from build123d import *

# Parameters (mm, degrees)
SKETCH1_W           = 300
SKETCH1_H           = 300
SKETCH1_W_2         = 350
BOSS_EXTRUDE1_DEPTH = 5
SKETCH2_W           = 50
SKETCH2_H           = 50
BOSS_EXTRUDE2_DEPTH = 75


with BuildPart() as part:
    # Sketch1 → Boss-Extrude1 (new body, symmetric)
    with BuildSketch(Plane(origin=(0, 0, 0), x_dir=(1, 0, 0), z_dir=(0, 1, 0))):
        Rectangle(SKETCH1_W, SKETCH1_H)
        with Locations((325, 0)):
            Rectangle(SKETCH1_W_2, SKETCH1_H)
    extrude(amount=BOSS_EXTRUDE1_DEPTH, both=True)

    # Sketch2 → Boss-Extrude2 (add)
    with BuildSketch(Plane(origin=(0, 5, 0), x_dir=(1, 0, 0), z_dir=(0, 1, 0))):
        with Locations((435, 0)):
            Rectangle(SKETCH2_W, SKETCH2_H)
    extrude(amount=BOSS_EXTRUDE2_DEPTH)


solid = part.part
CAD build for the part. Positions are in the model's coordinates, mm. A direction names the side the tool comes from. Coordinates: 2 decimals unless noted, no trailing zeros. Loops run counter-clockwise (first coordinate to the right, second up) from the corner with the lowest first, then second, coordinate; pieces in that order, holes last. Notation, with made-up numbers: (-4, 83) -> (44, 83) arc R21 ccw to (44, 109) -> close; hole circle Ø3 at (2, -25). An arc over 180 degrees is marked (long way). One line per item, written item: value.
1. Slice it at A-A on z = 2.5. Write the cut outline in (x, y), and give its area (4 significant figures).
Answers:
outline: (-150, -5) -> (500, -5) -> (500, 5) -> (460, 5) -> (460, 80) -> (410, 80) -> (410, 5) -> (-150, 5) -> close
area: 10,250 mm^2
2. Slice it at C-C on y = 29. Write the cut outline in (x, z).
Answers:
outline: (410, -25) -> (460, -25) -> (460, 25) -> (410, 25) -> close
3. Which spindle directions (+Z, -Z, +X, -X, +Y, -Y) get a long thin tool onto all of the face, cutting with end or side? Do faces 1 (the face through (410, 42, 0)), 2 (the face through (435, 42, -25)), 3 (the face through (435, 42, 25)), 4 (the face through (460, 42, 0)). Say none if no direction does.
Answers:
face 1: +Z, -Z, -X, +Y
face 2: -Z, +X, -X, +Y
face 3: +Z, +X, -X, +Y
face 4: +Z, -Z, +X, +Y
4. Slice it at B-B on x = 259. Write the cut outline in (y, z), and give its area (3 significant figures).
Answers:
outline: (-5, -150) -> (5, -150) -> (5, 150) -> (-5, 150) -> close
area: 3,000 mm^2
5. Flat gauge pins, fed straight in: P1, Ø8, axis at x = 411.5, y = 19.5, coming from the +Z side; P2, Ø3, axis at x = 118, z = 78.5, coming from the +Y side; P3, Ø8, axis at y = 36.5, z = 19, coming from the +X side. Where does each tip first touch, or does it go through?
Answers:
P1: stops at z = 25
P2: stops at y = 5
P3: stops at x = 460
6. Drill centre lines: line 1 (Y direction, x = 370, z = -42); line 2 (X direction, y = 26, z = 16); line 3 (Z direction, x = 419, y = 27). Where is each one in solid material? Low to high. Write a range as [from, to].
Answers:
line 1: y = [-5, 5]
line 2: x = [410, 460]
line 3: z = [-25, 25]
